Verification items for the finished model (mm, model axes). A direction names the side the tool comes from. Coordinates: 2 decimals unless noted, no trailing zeros. Order: outer loops, then holes, each group sorted by start corner. A loop starts at its lowest first (then second) coordinate and runs counter-clockwise, first axis right, second up. Notation, with made-up numbers: (-9, 9.5) -> (2, 9.5) arc R15 ccw to (2, 20.5) -> close; hole circle Ø4 at (46.25, 60.25). An arc over 180 degrees is marked (long way). Write item = value, one per line. Start each with the question number.
Autodesk Inventor part; units mm, degrees
ref_plane "YZ Plane" through (0, 0, 0) normal (1, 0, 0) x (0, 1, 0)
ref_plane "XZ Plane" through (0, 0, 0) normal (0, 1, 0) x (-1, 0, 0)
ref_plane "XY Plane" through (0, 0, 0) normal (0, 0, 1) x (1, 0, 0)
sketch "Sketch1" plane through (0, 0, 0) normal (0, 1, 0) x (-1, 0, 0)
  line L0 (8, 2) -> (-8, 2)
  line L1 (-8, 2) -> (-8, -2)
  line L2 (-8, -2) -> (8, -2)
  line L3 (8, -2) -> (8, 2)
  line L4 (11.2, 0) -> (-11.2, 0) construction
  line L5 (0, -2.8) -> (0, 2.8) construction
  point P0 (0, 0)
  dimension "d0" = 16
  dimension "d1" = 4
extrude "Extrusion1" add sketch "Sketch1" against normal blind 4.6
sketch "Sketch2" plane through (-8, 0, 2) normal (0, 0, 1) x (1, 0, 0)
  line L0 (6.8, -1.4) -> (9.2, -1.4)
  line L1 (9.2, -1.4) -> (9.2, -4.6)
  line L2 (9.2, -4.6) -> (6.8, -4.6)
  line L3 (6.8, -4.6) -> (6.8, -1.4)
  line L4 (16, -4.6) -> (0, -4.6)
  point P0 (8, 0)
  point P1 (8, -4.6)
  point P2 (8, -4.6)
  dimension "d4" = 2.4
  dimension "d5" = 3.2
extrude "Extrusion2" cut sketch "Sketch2" against normal through all
chamfer "Chamfer1" distance 1 angle 45 2 edges at (-1.2, -4.6, 0) (1.2, -4.6, 0)
fillet "Fillet1" radius 3 2 edges at (-8, -4.6, 0) (8, -4.6, 0)
sketch "Sketch3" plane through (0, 0, 0) normal (0, 1, 0) x (1, 0, 0)
  line L0 (-3, 0) -> (3, 0) construction
  line L1 (-3, -2.0001) -> (3, -2.0001)
  line L2 (3, 2.0001) -> (-3, 2.0001)
  arc A0 (-3, 2.0001) -> (-3, -2.0001) centre (-3, 0) ccw
  arc A1 (3, -2.0001) -> (3, 2.0001) centre (3, 0) ccw
  point P0 (0, 0)
  dimension "d12" = 3
extrude "Extrusion3" add sketch "Sketch3" along normal blind 1.5
sketch "Sketch4" plane through (0, 1.5, 0) normal (0, 1, 0) x (1, 0, 0)
  line L0 (-1.2, -2) -> (1.2, -2)
  line L1 (0.5, 2) -> (-0.5, 2)
  line L2 (-0.5, 2) -> (-0.5, -2)
  line L3 (-0.5, -2) -> (0.5, -2)
  line L4 (0.5, -2) -> (0.5, 2)
  line L5 (0.5, 2) -> (-0.5, -2) construction
  line L6 (-0.5, 2) -> (0.5, -2) construction
  point P0 (0, 0)
  dimension "d15" = 1
extrude "Extrusion4" add sketch "Sketch4" along normal blind 1.5
fillet "Fillet2" radius 2.8 2 edges at (0.5, 1.5, 0) (-0.5, 1.5, 0)
properties part number "Sliding_switch"
Item 1: Tool access check on faces 4 (the flat face through (-8, -1, 0)), 5 (the flat face through (-4, 1.5, 0)), 6 (the flat face through (1.7, -4.1, 0)). Record the directions out of +Z, -Z, +X, -X, +Y, -Y that give a thin tool (end or side, any length) a straight path to the whole face; none if there is none.
Item 2: Mould release check, pull along X, two halves, no side actions. Record for faces 1 (the flat face through (-7, 0, 0)), 2 (the cylindrical face through (-7.14, -3.7, 0.03)), 3 (the flat face through (1.2, -2, 0)): pulls with the +X half, pulls with the -X half, needs draft (parallel to the pull), parting line crosses it, or undercut.
Item 3: Gauge pin test, flat ends, axial feed: P1, Ø1.5, axis at x = 5.5, z = 0.5, coming from the +Y side; P2, Ø0.7, axis at y = -2.5, z = 0.5, coming from the +X side; P3, Ø0.7, axis at x = 0.5, z = -1, coming from the -Y side. Record the tip position at first contact, or that the pin passes through.
Item 4: Section check A-A (x = 0). Record the boundary of the cut face in (y, z), then the cut area to 3 significant figures.
Item 5: Section check C-C (y = -2). Record the boundary of the cut face in (x, z), then the cut area to 3 significant figures.
Item 6: Section check B-B (z = 0.85). Record the boundary of the cut face in (x, y), then the cut area to 3 significant figures.
Item 7: Thickness scan on line 1 (X direction, y = -1.5, z = 1.4); line 2 (Y direction, x = -5, z = 1.1); line 3 (X direction, y = -3.5, z = 0.35). Record the ranges inside material, lowest first.
Item 8: Section check D-D (x = -2.5). Record the boundary of the cut face in (y, z).
Filled sheet:
q1.face_4 = +Z, -Z, -X, +Y, -Y
q1.face_5 = +Z, -Z, -X, +Y
q1.face_6 = +Z, -Z, -Y
q2.face_1 = needs draft
q2.face_2 = pulls with the -X half
q2.face_3 = undercut
q3.P1 = 1.5
q3.P2 = 7.95
q3.P3 = -1.4
q4.outline = (-1.4, -2) -> (3, -2) -> (3, 2) -> (0, 2) -> (-1.4, 2) -> close
q4.area = 17.6 mm^2
q5.outline = (-7.97, -2) -> (-1.2, -2) -> (-1.2, 2) -> (-7.97, 2) -> close; (1.2, -2) -> (7.97, -2) -> (7.97, 2) -> (1.2, 2) -> close
q5.area = 54.2 mm^2
q6.outline = (-8, -1.6) arc R3 ccw to (-5, -4.6) -> (-2.2, -4.6) -> (-1.2, -3.6) -> (-1.2, -1.4) -> (1.2, -1.4) -> (1.2, -3.6) -> (2.2, -4.6) -> (5, -4.6) arc R3 ccw to (8, -1.6) -> (8, 0) -> (4.81, 0) -> (4.81, 1.5) -> (2.99, 1.5) arc R2.8 cw to (0.5, 3) -> (-0.5, 3) arc R2.8 cw to (-2.99, 1.5) -> (-4.81, 1.5) -> (-4.81, 0) -> (-8, 0) -> close
q6.area = 79.1 mm^2
q7.line_1 = -8 to -1.2, 1.2 to 8
q7.line_2 = -4.6 to 0
q7.line_3 = -7.32 to -1.2, 1.2 to 7.32
q8.outline = (-4.6, -2) -> (1.5, -2) -> (1.54, -2) -> (1.54, 2) -> (0, 2) -> (-4.6, 2) -> close
